The drawing under review shows one solid part. Ordinate dimensions are in mm from its lowest x, y, z. A direction names the side the tool comes from. Give positions to 0.01 mm unless a question says otherwise; leave off trailing zeros. Order: outer loops, then holes, each group sorted by start corner. A loop starts at its lowest first (then second) coordinate and runs counter-clockwise, first axis right, second up. Notation, with made-up numbers: (-8.75, 85.25) -> (2.25, 85.25) arc R15 ccw to (2.25, 96.25) -> close; hole circle Ø11 at (39, 71.25). An arc over 180 degrees is marked (long way). One line per item, written item: value.
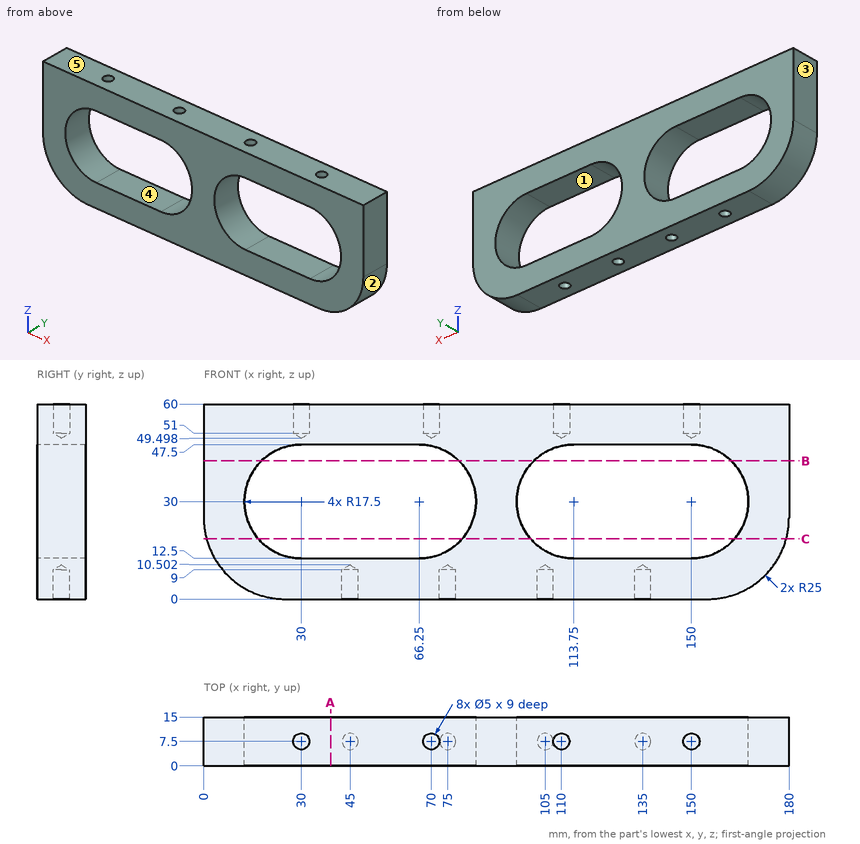
Item 1: Clearance check with flat-ended pins moving along their axes: P1, Ø4.5, axis at x = 45, y = 7.5, coming from the -Z side; P2, Ø3, axis at x = 110, y = 7.5, coming from the +Z side; P3, Ø12, axis at x = 108.5, z = 33.5, coming from the +Y side; P4, Ø6.5, axis at x = 70, y = 7.5, coming from the +Z side. State where each tip first meets the part, or that it passes through.
Returned:
P1: z = 9.15
P2: z = 50.4
P3: through
P4: z = 60
Item 2: Add section A-A on x = 39. Give the boundary of the cut face in (y, z).
Returned:
outline: (0, 0) -> (15, 0) -> (15, 12.5) -> (0, 12.5) -> close; (0, 47.5) -> (15, 47.5) -> (15, 60) -> (0, 60) -> close
Item 3: To check wall thickness, follow line 1 along X through (y, z) = (7.5, 56.5); line 2 along X through (y, z) = (2, 30); line 3 along Y through (x, z) = (70, 55). State the ranges of each line that lie inside material, in increasing order. Write a range as from..to.
Returned:
line 1: 0..27.5, 32.5..67.5, 72.5..107.5, 112.5..147.5, 152.5..180
line 2: 0..12.5, 83.75..96.25, 167.5..180
line 3: 0..5, 10..15
Item 4: Add section C-C on z = 18.5. Give the boundary of the cut face in (x, y).
Returned:
outline: (0.86, 0) -> (16.81, 0) -> (16.81, 15) -> (0.86, 15) -> close; (79.44, 0) -> (100.56, 0) -> (100.56, 15) -> (79.44, 15) -> close; (163.19, 0) -> (179.14, 0) -> (179.14, 15) -> (163.19, 15) -> close
Item 5: Add section B-B on z = 42.5. Give the boundary of the cut face in (x, y), plus the area to 3 significant figures.
Returned:
outline: (0, 0) -> (17.75, 0) -> (17.75, 15) -> (0, 15) -> close; (78.5, 0) -> (101.5, 0) -> (101.5, 15) -> (78.5, 15) -> close; (162.25, 0) -> (180, 0) -> (180, 15) -> (162.25, 15) -> close
area: 878 mm²
Item 6: Machinability: for the marked faces 1 and 2, which of the approach directions +Z, -Z, +X, -X, +Y, -Y give a long, thin tool a straight path to every point of the face, cutting with its end or side? Answer none if there is none.
Returned:
face 1: +Y, -Y
face 2: -Z, +X, +Y, -Y
Item 7: Draft analysis for pull direction Z (two halves, no side actions). For the marked faces 3, 4 and 5, state which applies: pulls with the +Z half, pulls with the -Z half, needs draft (parallel to the pull), parting line crosses it, or undercut.
Returned:
face 3: needs draft
face 4: undercut
face 5: pulls with the +Z half
